Design review of the part built by this model. Coordinates are the model's own, in mm. Face numbers are marked on the shaded views. Coordinates: 2 decimals unless noted, no trailing zeros. Write each loop counter-clockwise with the first axis right and the second up, starting at its lowest first coordinate (ties: lowest second). Pieces come first, ordered by that corner, then holes.
Q1. Take a section at A-A, the plane x = -34.5. Write out the cut boundary in (y, z), plus the area to 3 significant figures.
Q2. The part is to be moulded in two halves that separate along X. For the marked faces 1 and 2, say which applies: released by +X, released by -X, zero draft, split by the parting line, or undercut.
Q3. Take a section at B-B, the plane x = 5. Write out the cut boundary in (y, z).
Q4. Take a section at C-C, the plane z = -3. State how many separate pieces and enclosed holes the cut face has, plus the area to 3 significant figures.
Q5. For L1, parallel to Z at x = -18, y = 31.75; L2, parallel to Y at x = -5, z = -17; L3, parallel to X at y = 39, z = -50, list the stretches that pass through material, from the lowest coordinate up.
Q6. Take a section at D-D, the plane x = -14. Write out the cut boundary in (y, z), plus the area to 3 significant figures.
Q7. For pin 1 Ø2 at (x, y) = (-33.5, 39) entering from -Z; pin 2 Ø12 at (x, z) = (-38, -19) entering from -Y; pin 3 Ø2 at (x, y) = (21.5, 39) entering from +Z, all flat-tipped, find the tip position at first contact; note any pin that passes through.
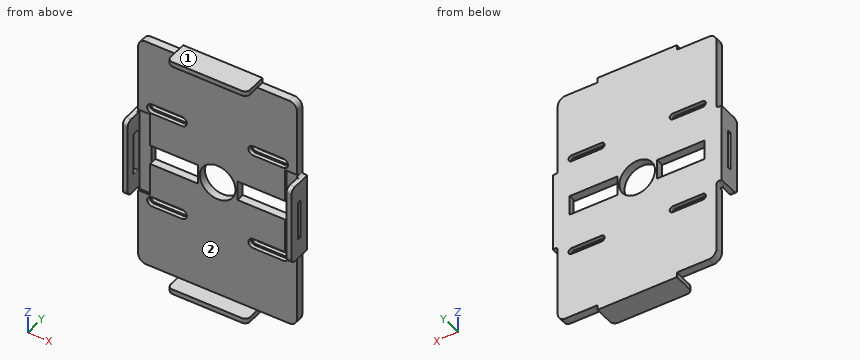
from build123d import *

# Parameters (mm, degrees)
SKETCH2_W                                 = 80
SKETCH2_H                                 = 120
SKETCH2_R                                 = 9
BOSS_EXTRUDE1_DEPTH                       = 4
FILLET1_R                                 = 4
BOSS_EXTRUDE3_START                       = -4
SKETCH3_W                                 = 40
SKETCH3_H                                 = 2.5
BOSS_EXTRUDE3_DEPTH                       = 12
FILLET5_R                                 = 2.5
FILLET5_OF_MIRROR6_R                      = 2.5
BOSS_EXTRUDE4_START                       = -4
SKETCH6_W                                 = 2.5
SKETCH6_H                                 = 39.999999999
BOSS_EXTRUDE4_DEPTH                       = 12
SKETCH13_W                                = 20
SKETCH13_H                                = 2
CUT_EXTRUDE6_DEPTH                        = 2.5
FILLET15_R                                = 1
FILLET15_OF_MIRROR31_R                    = 1
FILLET12_R                                = 1
FILLET9_R                                 = 2.5
SKETCH15_W                                = 24
SKETCH15_H                                = 10
CUT_EXTRUDE7_DEPTH                        = 4
SKETCH16_W                                = 43.464101615
SKETCH16_H                                = 1
CUT_EXTRUDE8_DEPTH                        = 6
CUT_EXTRUDE9_START                        = -2
CUT_EXTRUDE9_DEPTH                        = 2
MIRROR35_START                            = -2
MIRROR35_AT_THE_SECOND_PLANE_COPY_1_DEPTH = 2


with BuildPart() as part:
    # Sketch2 → Boss-Extrude1 (new body)
    with BuildSketch(Plane.XZ.offset(-40.230846757)):
        with Locations((-6.885042722, 0.192082071)):
            Rectangle(SKETCH2_W, SKETCH2_H)
        with Locations(Location((-6.885042722, 0.192082071, 0), (0, 0, 270))):
            Circle(SKETCH2_R, mode=Mode.SUBTRACT)
        with BuildLine():
            Line((-24.885042722, -26.407917929), (-39.885042722, -26.407917929))
            ThreePointArc((-39.885042722, -26.407917929), (-41.485042722, -24.807917929), (-39.885042722, -23.207917929))
            Line((-39.885042722, -23.207917929), (-24.885042722, -23.207917929))
            ThreePointArc((-24.885042722, -23.207917929), (-23.285042722, -24.807917929), (-24.885042722, -26.407917929))
        make_face(mode=Mode.SUBTRACT)
        with BuildLine():
            Line((-24.885042722, 23.592082071), (-39.885042722, 23.592082071))
            ThreePointArc((-39.885042722, 23.592082071), (-41.485042722, 25.192082071), (-39.885042722, 26.792082071))
            Line((-39.885042722, 26.792082071), (-24.885042722, 26.792082071))
            ThreePointArc((-24.885042722, 26.792082071), (-23.285042722, 25.192082071), (-24.885042722, 23.592082071))
        make_face(mode=Mode.SUBTRACT)
        with BuildLine():
            Line((26.114957278, 26.792082071), (11.114957278, 26.792082071))
            ThreePointArc((11.114957278, 26.792082071), (9.514957278, 25.192082071), (11.114957278, 23.592082071))
            Line((11.114957278, 23.592082071), (26.114957278, 23.592082071))
            ThreePointArc((26.114957278, 23.592082071), (27.714957278, 25.192082071), (26.114957278, 26.792082071))
        make_face(mode=Mode.SUBTRACT)
        with BuildLine():
            Line((26.114957278, -23.207917929), (11.114957278, -23.207917929))
            ThreePointArc((11.114957278, -23.207917929), (9.514957278, -24.807917929), (11.114957278, -26.407917929))
            Line((11.114957278, -26.407917929), (26.114957278, -26.407917929))
            ThreePointArc((26.114957278, -26.407917929), (27.714957278, -24.807917929), (26.114957278, -23.207917929))
        make_face(mode=Mode.SUBTRACT)
    extrude(amount=BOSS_EXTRUDE1_DEPTH)

    # Fillet1
    fillet1_edges = [part.edges().sort_by_distance(p)[0] for p in [
        (33.114957278, 38.230846757, -59.807917929),
        (-46.885042722, 38.230846757, -59.807917929),
        (-46.885042722, 38.230846757, 60.192082071),
        (33.114957278, 38.230846757, 60.192082071),
    ]]
    fillet(fillet1_edges, radius=FILLET1_R)

    # Sketch3 → Boss-Extrude3 (add)
    with BuildSketch(Plane.XZ.offset(-36.230846757).offset(BOSS_EXTRUDE3_START)):
        with Locations((-6.885042722, 61.442082071)):
            Rectangle(SKETCH3_W, SKETCH3_H)
    boss_extrude3 = extrude(amount=BOSS_EXTRUDE3_DEPTH)

    # Fillet5
    fillet5_edges = [part.edges().sort_by_distance(p)[0] for p in [
        (13.114957278, 28.230846757, 61.442082071),
        (-26.885042722, 28.230846757, 61.442082071),
    ]]
    fillet(fillet5_edges, radius=FILLET5_R)

    # Mirror6: Boss-Extrude3 across plane
    add(boss_extrude3.mirror(Plane(origin=(0, 0, 0.192082071), x_dir=(1, 0, 0), z_dir=(0, 0, -1))))

    # Fillet5 of Mirror6
    fillet5_of_mirror6_edges = [part.edges().sort_by_distance(p)[0] for p in [
        (13.114957278, 28.230846757, -61.057917929),
        (-26.885042722, 28.230846757, -61.057917929),
    ]]
    fillet(fillet5_of_mirror6_edges, radius=FILLET5_OF_MIRROR6_R)

    # Sketch6 → Boss-Extrude4 (add)
    with BuildSketch(Plane.XZ.offset(-36.230846757).offset(BOSS_EXTRUDE4_START)):
        with Locations((-48.135042722, 0.19208207)):
            Rectangle(SKETCH6_W, SKETCH6_H)
    boss_extrude4 = extrude(amount=BOSS_EXTRUDE4_DEPTH)

    # Sketch13 → Cut-Extrude6 (cut)
    with BuildSketch(Plane.ZY.offset(49.385042722)):
        with Locations((0.192082071, 34.230846757)):
            Rectangle(SKETCH13_W, SKETCH13_H)
    cut_extrude6 = extrude(amount=-CUT_EXTRUDE6_DEPTH, mode=Mode.SUBTRACT)

    # Fillet15
    fillet15_edges = [part.edges().sort_by_distance(p)[0] for p in [
        (-46.885042722, 35.230846757, 0.192082071),
        (-46.885042722, 34.230846757, -9.807917929),
        (-46.885042722, 33.230846757, 0.192082071),
        (-46.885042722, 34.230846757, 10.192082071),
    ]]
    fillet(fillet15_edges, radius=FILLET15_R - 0.0001)  # a hair under: the kernel refuses the full size

    # Mirror31: Boss-Extrude4, Cut-Extrude6 across plane
    add(boss_extrude4.mirror(Plane.ZY.offset(6.885042722)))
    add(cut_extrude6.mirror(Plane.ZY.offset(6.885042722)), mode=Mode.SUBTRACT)

    # Fillet15 of Mirror31
    fillet15_of_mirror31_edges = [part.edges().sort_by_distance(p)[0] for p in [
        (33.114957278, 35.230846757, 0.192082071),
        (33.114957278, 34.230846757, -9.807917929),
        (33.114957278, 33.230846757, 0.192082071),
        (33.114957278, 34.230846757, 10.192082071),
    ]]
    fillet(fillet15_of_mirror31_edges, radius=FILLET15_OF_MIRROR31_R - 0.0001)  # a hair under: the kernel refuses the full size

    # Fillet12
    fillet12_edges = [part.edges().sort_by_distance(p)[0] for p in [
        (-46.885042722, 38.230846757, 20.19208207),
        (-46.885042722, 38.230846757, -19.807917929),
        (33.114957278, 38.230846757, -19.807917929),
        (33.114957278, 38.230846757, 20.19208207),
    ]]
    fillet(fillet12_edges, radius=FILLET12_R)

    # Fillet9
    fillet9_edges = [part.edges().sort_by_distance(p)[0] for p in [
        (-48.135042722, 28.230846757, -19.807917929),
        (-48.135042722, 28.230846757, 20.19208207),
        (34.364957278, 28.230846757, -19.807917929),
        (34.364957278, 28.230846757, 20.19208207),
    ]]
    fillet(fillet9_edges, radius=FILLET9_R)

    # Sketch15 → Cut-Extrude7 (cut)
    with BuildSketch(Plane(origin=(0, 40.230846757, 0), x_dir=(1, 0, 0), z_dir=(0, 1, 0))):
        with Locations((15.114957278, -0.192082071)):
            Rectangle(SKETCH15_W, SKETCH15_H)
    cut_extrude7 = extrude(amount=-CUT_EXTRUDE7_DEPTH, mode=Mode.SUBTRACT)

    # Mirror32: Cut-Extrude7 across plane
    add(cut_extrude7.mirror(Plane.ZY.offset(6.885042722)), mode=Mode.SUBTRACT)

    # Sketch16 → Cut-Extrude8 (cut)
    with BuildSketch(Plane.ZY.offset(46.885042722)):
        with Locations((0.19208207, 36.730846757)):
            Rectangle(SKETCH16_W, SKETCH16_H)
    cut_extrude8 = extrude(amount=-CUT_EXTRUDE8_DEPTH, mode=Mode.SUBTRACT)

    # Mirror34: Cut-Extrude8 across plane
    add(cut_extrude8.mirror(Plane.ZY.offset(6.885042722)), mode=Mode.SUBTRACT)

    # Sketch17 → Cut-Extrude9 (cut)
    with BuildSketch(Plane.XZ.offset(-36.230846757).offset(CUT_EXTRUDE9_START)):
        with BuildLine():
            Line((-39.885042722, 22.692082071), (-24.885042722, 22.692082071))
            ThreePointArc((-24.885042722, 22.692082071), (-22.385042722, 25.192082071), (-24.885042722, 27.692082071))
            Line((-24.885042722, 27.692082071), (-39.885042722, 27.692082071))
            ThreePointArc((-39.885042722, 27.692082071), (-42.385042722, 25.192082071), (-39.885042722, 22.692082071))
        make_face()
        with BuildLine():
            Line((-39.885042722, 23.592082071), (-24.885042722, 23.592082071))
            ThreePointArc((-24.885042722, 23.592082071), (-23.285042722, 25.192082071), (-24.885042722, 26.792082071))
            Line((-24.885042722, 26.792082071), (-39.885042722, 26.792082071))
            ThreePointArc((-39.885042722, 26.792082071), (-41.485042722, 25.192082071), (-39.885042722, 23.592082071))
        make_face(mode=Mode.SUBTRACT)
    cut_extrude9 = extrude(amount=CUT_EXTRUDE9_DEPTH, mode=Mode.SUBTRACT)

    # Mirror35: Cut-Extrude9 across plane
    add(cut_extrude9.mirror(Plane(origin=(0, 0, 0.192082071), x_dir=(1, 0, 0), z_dir=(0, 0, -1))), mode=Mode.SUBTRACT)

    # Mirror35 at the second plane: Cut-Extrude9 across plane
    add(cut_extrude9.mirror(Plane.ZY.offset(6.885042722)), mode=Mode.SUBTRACT)

    # Mirror35 at the second plane copy 1 sket → Mirror35 at the second plane copy 1 (cut)
    with BuildSketch(Plane(origin=(-13.770085443, 36.230846757, 0.384164141), x_dir=(-1, 0, 0), z_dir=(0, -1, 0)).offset(MIRROR35_START)):
        with BuildLine():
            Line((-39.885042722, 22.692082071), (-24.885042722, 22.692082071))
            ThreePointArc((-24.885042722, 22.692082071), (-22.385042722, 25.192082071), (-24.885042722, 27.692082071))
            Line((-24.885042722, 27.692082071), (-39.885042722, 27.692082071))
            ThreePointArc((-39.885042722, 27.692082071), (-42.385042722, 25.192082071), (-39.885042722, 22.692082071))
        make_face()
        with BuildLine():
            Line((-39.885042722, 23.592082071), (-24.885042722, 23.592082071))
            ThreePointArc((-24.885042722, 23.592082071), (-23.285042722, 25.192082071), (-24.885042722, 26.792082071))
            Line((-24.885042722, 26.792082071), (-39.885042722, 26.792082071))
            ThreePointArc((-39.885042722, 26.792082071), (-41.485042722, 25.192082071), (-39.885042722, 23.592082071))
        make_face(mode=Mode.SUBTRACT)
    extrude(amount=MIRROR35_AT_THE_SECOND_PLANE_COPY_1_DEPTH, mode=Mode.SUBTRACT)


solid = part.part
Responses:
1. outline: (36.23, -59.81) - (40.23, -59.81) - (40.23, -26.41) - (38.23, -26.41) - (38.23, -27.31) - (36.23, -27.31) - close; (36.23, -22.31) - (38.23, -22.31) - (38.23, -23.21) - (40.23, -23.21) - (40.23, -4.81) - (36.23, -4.81) - close; (36.23, 5.19) - (40.23, 5.19) - (40.23, 23.59) - (38.23, 23.59) - (38.23, 22.69) - (36.23, 22.69) - close; (36.23, 27.69) - (38.23, 27.69) - (38.23, 26.79) - (40.23, 26.79) - (40.23, 60.19) - (36.23, 60.19) - close
1. area: 407 mm2
2. face 1: zero draft
2. face 2: undercut
3. outline: (28.23, -62.31) - (40.23, -62.31) - (40.23, -4.81) - (36.23, -4.81) - (36.23, -59.81) - (28.23, -59.81) - close; (28.23, 60.19) - (36.23, 60.19) - (36.23, 5.19) - (40.23, 5.19) - (40.23, 62.69) - (28.23, 62.69) - close
4. separate pieces: 6
4. enclosed holes: 0
4. area: 97.8 mm2
5. L1: z = -62.31 to -59.81, 60.19 to 62.69
5. L2: y = 36.23 to 40.23
5. L3: x = -46.89 to 33.11
6. outline: (28.23, -62.31) - (40.23, -62.31) - (40.23, -5.32) - (36.23, -5.32) - (36.23, -59.81) - (28.23, -59.81) - close; (28.23, 60.19) - (36.23, 60.19) - (36.23, 5.7) - (40.23, 5.7) - (40.23, 62.69) - (28.23, 62.69) - close
6. area: 496 mm2
7. pin 1: stops at z = -59.81
7. pin 2: stops at y = 36.23
7. pin 3: stops at z = 60.19
